Job drawing, mm, ordinate dimensions from the low corner. One solid piece. A direction names the side the tool comes from. Give positions to 0.01 mm unless a question says otherwise; leave off trailing zeros. Order: outer loops, then holes, each group sorted by start corner. A loop starts at its lowest first (then second) coordinate and runs counter-clockwise, first axis right, second up. Notation, with made-up numbers: M 36,-37.75 L 78,-37.75 A23 cw 78,-23.75 Z; hole C 79,-3.75 d6. An arc over 180 degrees is marked long. One line per question, with ' | ' between items.
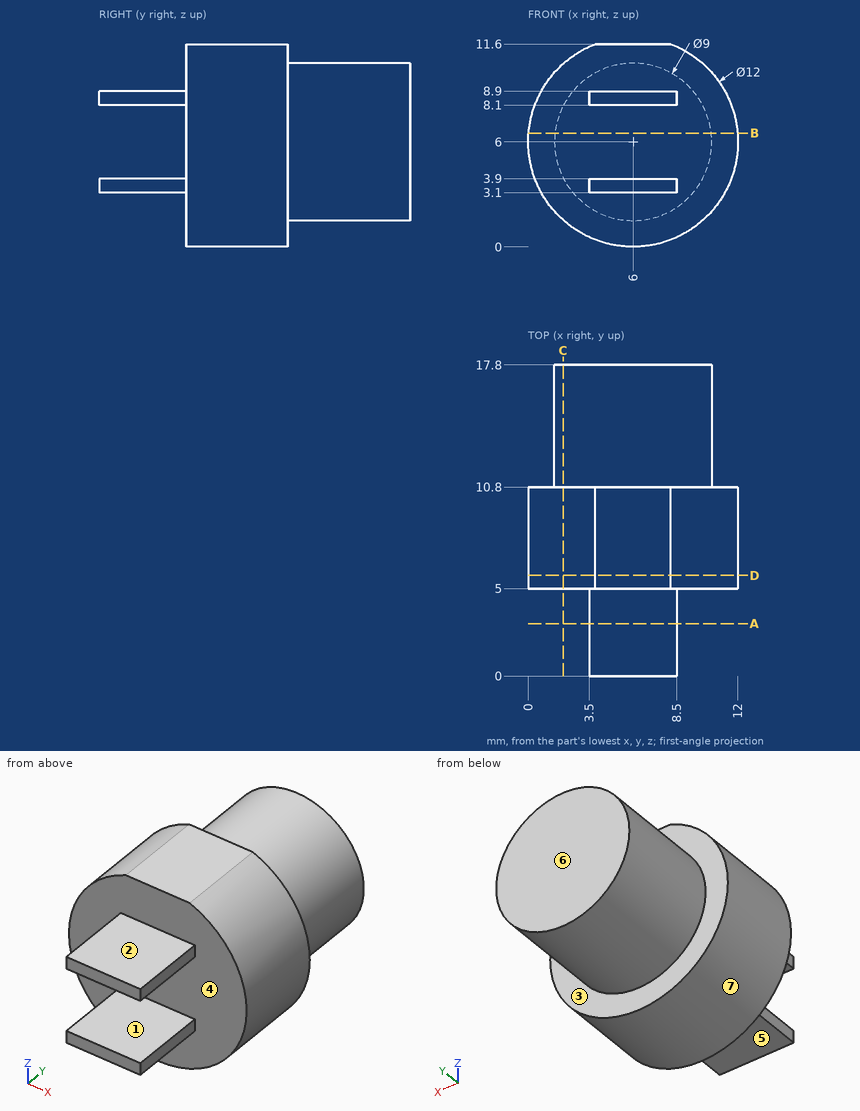
1. Slice it at B-B on z = 6.5. Give the cut face in (x, y).
Worked out:
outline: M 0.02,5 L 11.98,5 L 11.98,10.8 L 10.47,10.8 L 10.47,17.8 L 1.53,17.8 L 1.53,10.8 L 0.02,10.8 Z
2. Probe L1, parallel to Z at x = 3.75, y = 2.75; L2, parallel to Y at x = 2.75, z = 1.5; L3, parallel to Y at x = 2.5, z = 6.5. List the from-to ranges inside material, lowest first. Write a range as from..to.
Worked out:
L1: z = 3.1..3.9, 8.1..8.9 | L2: y = 5..10.8 | L3: y = 5..17.8
3. Slice it at D-D on y = 5.75. Give the cut face in (x, z), then the cut area to 3 significant figures.
Worked out:
outline: M 3.85,11.6 A6 ccw long 8.15,11.6 Z | area: 112 mm2
4. Drop flat-ended pins along their axis: pin 1 (2.5 mm diameter, centred on x = 6, y = 3.5, fed in from +Z); pin 2 (0.6 mm diameter, centred on y = 1.5, z = 8.5, fed in from -X); pin 3 (5 mm diameter, centred on y = 4.5, z = 7.5, fed in from -X); pin 4 (4 mm diameter, centred on x = 7, y = 2.5, fed in from -Z). Give the stop position or say it passes through.
Worked out:
pin 1: stops at z = 8.9 | pin 2: stops at x = 3.5 | pin 3: stops at x = 0 | pin 4: stops at z = 3.1
5. Tool access for the marked faces 1, 2 and 3: list every direction of +Z, -Z, +X, -X, +Y, -Y with a clear straight run to the whole face (end or side of a thin tool).
Worked out:
face 1: +X, -X, -Y | face 2: +Z, +X, -X, -Y | face 3: +Y
6. Slice it at C-C on x = 2. Give the cut face in (y, z).
Worked out:
outline: M 5,1.53 L 10.8,1.53 L 10.8,3.94 L 17.8,3.94 L 17.8,8.06 L 10.8,8.06 L 10.8,10.47 L 5,10.47 Z
7. Slice it at A-A on y = 3. Give the cut face in (x, z), then the cut area to 3 significant figures.
Worked out:
outline: M 3.5,3.1 L 8.5,3.1 L 8.5,3.9 L 3.5,3.9 Z; M 3.5,8.1 L 8.5,8.1 L 8.5,8.9 L 3.5,8.9 Z | area: 8.00 mm2
8. Mould opens along Z. For the marked faces 4, 5, 6 and 7 say: released by +Z, released by -Z, zero draft, split by the parting line, or undercut.
Worked out:
face 4: undercut | face 5: released by -Z | face 6: zero draft | face 7: split by the parting line
